Here's how the part is built. I have some questions about the finished solid (model axes, mm). Face numbers are marked on the shaded views. Coordinates: 2 decimals unless noted, no trailing zeros. Write each loop counter-clockwise with the first axis right and the second up, starting at its lowest first coordinate (ties: lowest second). Pieces come first, ordered by that corner, then holes.
(1) Imagine slicing it at B-B, the plane z = 9.5. List the corners of the cut face in (x, y) for me, plus the area to 3 significant figures.
(2) For pin 1 Ø2.5 at (x, z) = (-8.75, -8.75) entering from +Y, with a flat end and sliding along its axis, tell me the tip position at first contact or that it passes through.
(3) Imagine slicing it at A-A, the plane y = 2.2. List the corners of the cut face in (x, z) for me.
(4) Thinking about a two-plate mould opening in X: for the marked faces 1, 2 and 3, which applies, released by +X, released by -X, zero draft, split by the parting line, or undercut?
(5) Please list where these lines run through material, in increasing order: probe 1 along Z at (x, y) = (-8.75, 2.4); probe 2 along X at (y, z) = (1.8, 8.75); probe 3 along Z at (x, y) = (-9.75, 1.9).
```python
from build123d import *

# Parameters (mm, degrees)
ESQUISSE1_W        = 24
ESQUISSE1_H        = 24
BOSS_EXTRU_1_DEPTH = 4
D_GAGEMENT_M31_D   = 3.4
CONG_1_R           = 3


with BuildPart() as part:
    # Esquisse1 → Boss.-Extru.1 (new body)
    with BuildSketch(Plane(origin=(0, 0, 0), x_dir=(1, 0, 0), z_dir=(0, 1, 0))):
        Rectangle(ESQUISSE1_W, ESQUISSE1_H)
    extrude(amount=BOSS_EXTRU_1_DEPTH)

    # Dégagement M31 (through all)
    with Locations(Plane(origin=(0, 4, 0), x_dir=(1, 0, 0), z_dir=(0, 1, 0))):
        with Locations((-8.75, -8.75), (-8.75, 8.75)):
            Hole(D_GAGEMENT_M31_D / 2)

    # Congé1
    cong_1_edges = [part.edges().sort_by_distance(p)[0] for p in [
        (12, 2, 12),
        (-12, 2, 12),
        (-12, 2, -12),
        (12, 2, -12),
    ]]
    fillet(cong_1_edges, radius=CONG_1_R)


solid = part.part
```
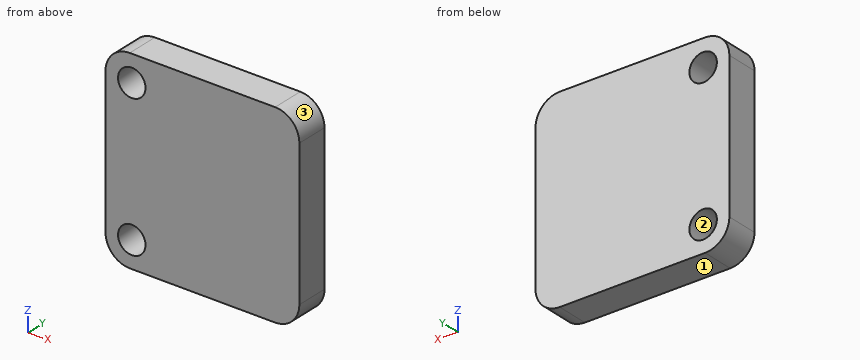
Recorded:
1. outline: (-11.96, 0) - (-10.28, 0) - (-10.28, 4) - (-11.96, 4) - close; (-7.22, 0) - (11.96, 0) - (11.96, 4) - (-7.22, 4) - close
1. area: 83.5 mm2
2. pin 1: passes through
3. outline: (-12, -9) arc R3 ccw to (-9, -12) - (9, -12) arc R3 ccw to (12, -9) - (12, 9) arc R3 ccw to (9, 12) - (-9, 12) arc R3 ccw to (-12, 9) - close; hole circle Ø3.4 at (-8.75, -8.75); hole circle Ø3.4 at (-8.75, 8.75)
4. face 1: zero draft
4. face 2: undercut
4. face 3: released by +X
5. probe 1: z = -12 to -10.45, -7.05 to 7.05, 10.45 to 12
5. probe 2: x = -12 to -10.45, -7.05 to 12
5. probe 3: z = -11.9 to -10.12, -7.38 to 7.38, 10.12 to 11.9
